Source: three-view drawing plus pictorial views. Frame: mm from the lowest corner of the part. Round coordinates to 2 decimals unless told otherwise and drop trailing zeros. Loops run counter-clockwise (first coordinate to the right, second up) from the corner with the lowest first, then second, coordinate; pieces in that order, holes last. Notation, with made-up numbers: (21, 73) -> (75, 73) arc R23 ccw to (75, 103) -> close; hole circle Ø5 at (71, 26.25). An arc over 180 degrees is marked (long way). One line per question, with ' | ' between items. Start each with the question number.
Q1. Cut plane A-A on x = 5. Return loops of the section in (y, z), and give its area (3 significant figures).
Q2. Material intervals for L1, parallel to Z at x = 5.25, y = 0.55 (3 decimals); L2, parallel to Z at x = 5, y = 1.2; L3, parallel to Z at x = 8, y = 0.4, sorted ascending.
Q3. Cut plane B-B on y = 2. Return loops of the section in (x, z).
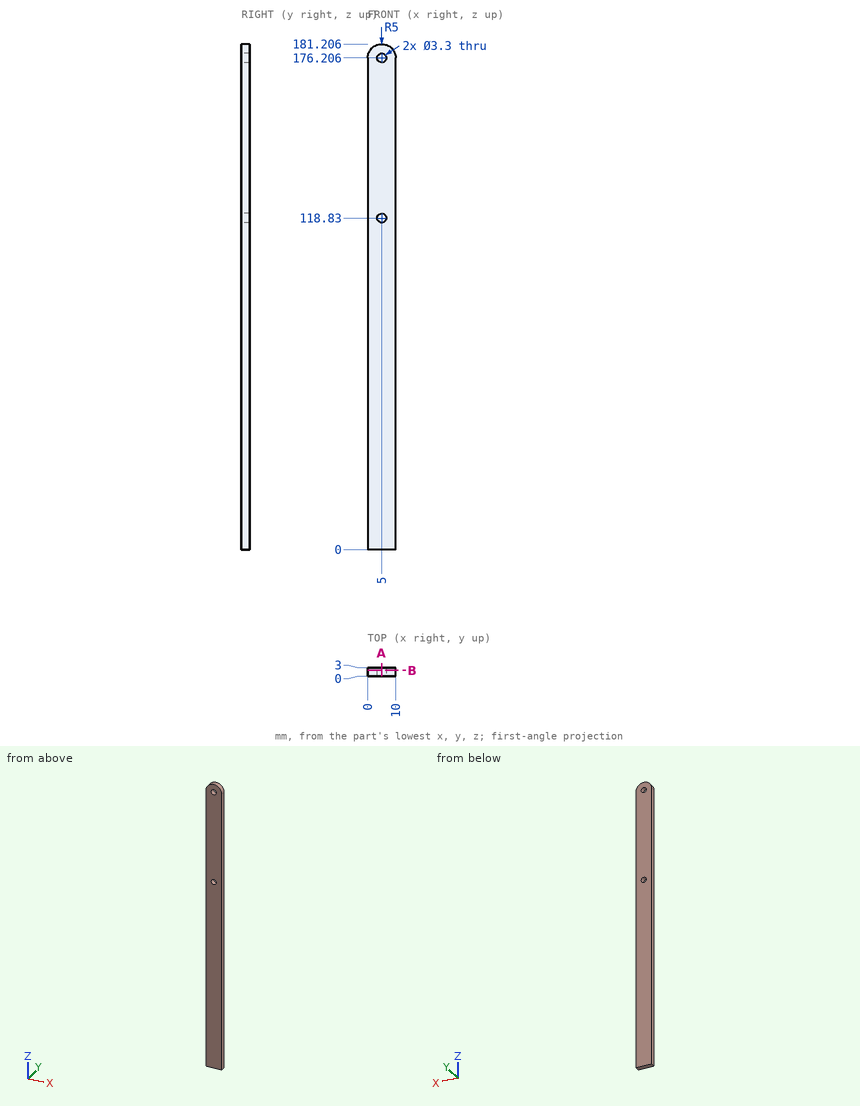
Results:
1) outline: (0, 0) -> (3, 0) -> (3, 117.18) -> (0, 117.18) -> close; (0, 120.48) -> (3, 120.48) -> (3, 174.56) -> (0, 174.56) -> close; (0, 177.86) -> (3, 177.86) -> (3, 181.21) -> (0, 181.21) -> close | area: 524 mm^2
2) L1: 0 to 117.199, 120.461 to 174.575, 177.837 to 181.2 | L2: 0 to 117.18, 120.48 to 174.56, 177.86 to 181.21 | L3: 0 to 180.21
3) outline: (0, 0) -> (10, 0) -> (10, 176.21) arc R5 ccw to (0, 176.21) -> close; hole circle Ø3.3 at (5, 118.83); hole circle Ø3.3 at (5, 176.21)
